CAD build for the part. Positions are in the model's coordinates, mm. Face numbers are marked on the shaded views. A direction names the side the tool comes from. Round coordinates to 2 decimals unless told otherwise and drop trailing zeros. Loops run counter-clockwise (first coordinate to the right, second up) from the corner with the lowest first, then second, coordinate; pieces in that order, holes last. Notation, with made-up numbers: M 8.25,29.5 L 12.25,29.5 A9 cw 12.25,33.5 Z; hole C 28.25,46 d5. An arc over 180 degrees is marked long. One line per item, written item: value. Start each with the question number.
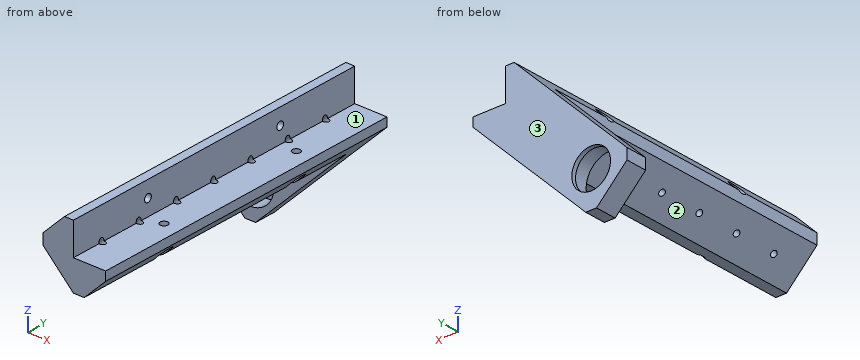
Autodesk Inventor part; units mm, degrees
ref_plane "YZ Plane" through (0, 0, 0) normal (1, 0, 0) x (0, 1, 0)
ref_plane "XZ Plane" through (0, 0, 0) normal (0, 1, 0) x (-1, 0, 0)
ref_plane "XY Plane" through (0, 0, 0) normal (0, 0, 1) x (1, 0, 0)
sketch "Sketch1" plane through (0, 0, 0) normal (0, 1, 0) x (-1, 0, 0)
  line L0 (0, 0) -> (0, 15)
  line L1 (0, 15) -> (14.1421, 15)
  line L2 (14.1421, 15) -> (14.1421, 0)
  line L3 (14.1421, 0) -> (0, -14.1421)
  line L4 (0, -14.1421) -> (-15, -14.1421)
  line L5 (-15, -14.1421) -> (-15, 0)
  line L6 (-15, 0) -> (0, 0)
  dimension "d0" = 15
  dimension "d1" = 10
extrude "Extrusion1" add sketch "Sketch1" along normal blind 151
chamfer "Chamfer1" distance 10 angle 45 2 edges at (-14.1421, 75.5, 15) (15, 75.5, -14.1421)
sketch "Sketch2" plane through (0, 151, 0) normal (0, 1, 0) x (1, 0, 0)
  line L0 (5, 14.1421) -> (15, 4.1421)
  line L1 (5, 14.1421) -> (0, 14.1421)
  line L2 (0, 14.1421) -> (-14.1421, 0)
  line L3 (-14.1421, 0) -> (-14.1421, -5)
  line L4 (-4.1421, -15) -> (-14.1421, -5)
  line L5 (-4.1421, -15) -> (0, -15)
  line L6 (0, -15) -> (0, 0)
  line L7 (0, 0) -> (15, 0)
  line L8 (15, 0) -> (15, 4.1421)
  circle A0 centre (-39.9264, 39.9264) radius 11
  line L9 (5, 14.1421) -> (-37.4264, 56.5685)
  line L10 (-37.4264, 56.5685) -> (-42.4264, 56.5685)
  line L11 (-42.4264, 56.5685) -> (-56.5685, 42.4264)
  line L12 (-56.5685, 42.4264) -> (-56.5685, 37.4264)
  line L13 (-56.5685, 37.4264) -> (-14.1421, -5)
  line L14 (-4.1421, -15) -> (-14.1421, -5)
  line L15 (5, 14.1421) -> (15, 4.1421)
  line L16 (-14.1421, 0) -> (-14.1421, -5)
  dimension "d7" = 22
  dimension "d8" = 60
  dimension "d9" = 27.0711
  dimension "d10" = 13.5355
  dimension "d11" = 13.5355
extrude "Extrusion2" add sketch "Sketch2" against normal blind 10 contours L1 L2 L3 L13 L12 L11 L10 L9
sketch "Sketch3" plane through (0, 151, 0) normal (0, 1, 0) x (1, 0, 0)
  circle A0 centre (-39.9264, 39.9264) radius 11
  circle A1 centre (-39.9264, 39.9264) radius 9
  point P0 (0, 0)
  dimension "d14" = 2
extrude "Extrusion3" add sketch "Sketch3" against normal blind 2
sketch "Sketch4" plane through (-14.1421, 0, 0) normal (-1, 0, 0) x (0, 0, 1)
  line L0 (5, 141) -> (0, 141)
  line L1 (0, 0) -> (0, 141)
  line L2 (0, 0) -> (5, 0)
  line L3 (5, 141) -> (5, 0)
  line L4 (-37.4264, 151) -> (15, 151)
  line L5 (-37.4264, 151) -> (-37.4264, 141)
  line L6 (5, 141) -> (-37.4264, 141)
  line L7 (5, 141) -> (5, 0)
  line L8 (5, 0) -> (15, 0)
  line L9 (15, 0) -> (15, 151)
  point P0 (0, 0)
  point P1 (7.5, 40)
  point P2 (7.5, 111)
  dimension "d17" = 7.5
  dimension "d18" = 40
  dimension "d19" = 40
hole "Hole1" at (-14.1421, 40, 7.5) at (-14.1421, 111, 7.5) direction (1, 0, 0) diameter 3.6 end through all counterbore diameter 6.5 counterbore depth 10
sketch "Sketch5" plane through (5, 0, -14.1421) normal (0, 0, -1) x (-1, 0, 0)
  line L0 (5, 141) -> (0, 141)
  line L1 (0, 0) -> (0, 141)
  line L2 (0, 0) -> (5, 0)
  line L3 (5, 0) -> (5, 141)
  line L4 (-10, 151) -> (42.4264, 151)
  line L5 (-10, 151) -> (-10, 0)
  line L6 (-10, 0) -> (0, 0)
  line L7 (0, 0) -> (0, 141)
  line L8 (42.4264, 141) -> (0, 141)
  line L9 (42.4264, 151) -> (42.4264, 141)
  point P0 (-2.5, 40)
  point P1 (-2.5, 111)
  dimension "d27" = 7.5
  dimension "d28" = 40
  dimension "d29" = 40
hole "Hole2" at (7.5, 40, -14.1421) at (7.5, 111, -14.1421) direction (0, 0, 1) diameter 3.6 end through all counterbore diameter 6.5 counterbore depth 10
sketch "Sketch6" plane through (0, 0, -14.1421) normal (-0.7071, 0, -0.7071) x (-0.7071, 0, 0.7071)
  circle A0 centre (10, -125) radius 3
  circle A1 centre (10, -85) radius 3
  circle A2 centre (10, -45) radius 3
  circle A3 centre (10, -5) radius 3
  circle A4 centre (10, 35) radius 3
  circle A5 centre (10, 75) radius 3
  circle A6 centre (10, 115) radius 3
  circle A7 centre (10, 135) radius 3
  circle A8 centre (10, 95) radius 3
  circle A9 centre (10, 55) radius 3
  circle A10 centre (10, 15) radius 3
  circle A11 centre (10, -25) radius 3
  circle A12 centre (10, -65) radius 3
  circle A13 centre (10, -105) radius 3
  circle A14 centre (10, -145) radius 3
  line L0 (14.5, 140) -> (5.5, 140)
  line L1 (5.5, 140) -> (5.5, -210)
  line L2 (14.5, -210) -> (5.5, -210)
  line L3 (14.5, 140) -> (14.5, -210)
  circle A15 centre (10, -205) radius 3
  circle A16 centre (10, -165) radius 3
  circle A17 centre (10, -185) radius 3
  point P0 (10, 0)
hole "Hole3" at (-7.0711, 15, -7.0711) at (-7.0711, 35, -7.0711) at (-7.0711, 55, -7.0711) at (-7.0711, 75, -7.0711) at (-7.0711, 95, -7.0711) at (-7.0711, 115, -7.0711) at (-7.0711, 135, -7.0711) direction (0.7071, 0, 0.7071) diameter 2.8 end through all
equation "\"d10\" = 0.5 * d9"
equation "\"d11\" = d10"
properties part number "Corner Z Brace w Bearing" material "ABS Plastic"
(1) Flat gauge pins, fed straight in: P1, Ø8.5, axis at x = 7.5, y = 40, coming from the +Z side; P2, Ø4, axis at y = 50.5, z = 3, coming from the -X side; P3, Ø12, axis at x = -45.5, z = -41.5, coming from the -Y side. Where does each tip first touch, or does it go through?
(2) Slice it at C-C, the plane y = 111. List the corners of the cut face in (x, z), and give its area (3 significant figures).
(3) Probe L1, parallel to Y at x = 7.5, z = -8; L2, parallel to Y at x = -28, z = -26; L3, parallel to Z at x = -2.1, y = 40. List the from-to ranges inside material, lowest first.
(4) Slice it at D-D, the plane x = -45. List the corners of the cut face in (y, z), and give its area (3 significant figures).
(5) Which spindle directions (+Z, -Z, +X, -X, +Y, -Y) get a long thin tool onto all of the face, cutting with end or side? Do the marked faces 1, 2 and 3. Say none if no direction does.
(6) Slice it at B-B, the plane z = 7.5. List the corners of the cut face in (x, y).
(7) Slice it at A-A, the plane x = 7.5. List the corners of the cut face in (y, z).
Check result:
1. P1: stops at z = 0
1. P2: stops at x = -14.14
1. P3: stops at y = 141
2. outline: M -14.14,0 L 0,-14.14 L 4.25,-14.14 L 4.25,-4.14 L 5.7,-4.14 L 5.7,0 L 0,0 L 0,5.7 L -4.14,5.7 L -4.14,4.25 L -14.14,4.25 Z; M -8.39,10.75 L -4.14,10.75 L -4.14,9.3 L 0,9.3 L 0,15 L -4.14,15 Z; M 9.3,-4.14 L 10.75,-4.14 L 10.75,-8.39 L 15,-4.14 L 15,0 L 9.3,0 Z
2. area: 298 mm^2
3. L1: y = 0 to 36.75, 43.25 to 107.75, 114.25 to 151
3. L2: y = 141 to 151
3. L3: z = -12.04 to 5.7, 9.3 to 15
4. outline: M 141,-53.99 L 151,-53.99 L 151,-47.36 L 149,-47.36 L 149,-49.69 L 141,-49.69 Z; M 141,-30.17 L 149,-30.17 L 149,-32.49 L 151,-32.49 L 151,-25.86 L 141,-25.86 Z
4. area: 95.5 mm^2
5. face 1: +Z, +X, +Y, -Y
5. face 2: -Z, -X, -Y
5. face 3: +Z, -Z, +X, -X, +Y
6. outline: M -11.64,0 L 0,0 L 0,38.2 L -4.14,38.2 L -4.14,36.75 L -11.64,36.75 Z; M -11.64,43.25 L -4.14,43.25 L -4.14,41.8 L 0,41.8 L 0,109.2 L -4.14,109.2 L -4.14,107.75 L -11.64,107.75 Z; M -11.64,114.25 L -4.14,114.25 L -4.14,112.8 L 0,112.8 L 0,151 L -11.64,151 Z
7. outline: M 0,-11.64 L 36.75,-11.64 L 36.75,-4.14 L 38.2,-4.14 L 38.2,0 L 0,0 Z; M 41.8,-4.14 L 43.25,-4.14 L 43.25,-11.64 L 107.75,-11.64 L 107.75,-4.14 L 109.2,-4.14 L 109.2,0 L 41.8,0 Z; M 112.8,-4.14 L 114.25,-4.14 L 114.25,-11.64 L 151,-11.64 L 151,0 L 112.8,0 Z
